Read the model definition and answer for the solid it produces. Units are mm, in the model's axes. Coordinates: 2 decimals unless noted, no trailing zeros. Order: outer loops, then holes, each group sorted by start corner. A loop starts at its lowest first (then second) coordinate and runs counter-clockwise, first axis right, second up. Notation, with made-up numbers: M -25,35 L 7,35 A31 cw 7,74 Z; hole C -28,57 d7. An arc over 180 degrees is marked long. Put each result on its own line as item: value.
from build123d import *

# Parameters (mm, degrees)
F0_R     = 17.5
F1_DEPTH = 11
F2_R     = 7.5
F3_DEPTH = 11.001
F4_R     = 0.5
F5_R     = 0.5


with BuildPart() as f1:
    # F0 (on Top) → F1 (new body)
    with BuildSketch(Plane.XY):
        Circle(F0_R)
    extrude(amount=F1_DEPTH)

    # F2 (on face) → F3 (cut, through all)
    with BuildSketch(Plane.XY.offset(11)):
        Circle(F2_R)
    extrude(amount=-F3_DEPTH, mode=Mode.SUBTRACT)

    # F4
    f4_edges = [f1.edges().sort_by_distance(p)[0] for p in [
        (-17.5, 0, 11),
        (-17.5, 0, 0),
    ]]
    fillet(f4_edges, radius=F4_R)

    # F5
    f5_edges = [f1.edges().sort_by_distance(p)[0] for p in [
        (-7.5, 0, 11),
        (-7.5, 0, 0),
    ]]
    fillet(f5_edges, radius=F5_R)


solid = f1.part
Q1. Find section A-A on x = 0. Write down the section's boundary in (y, z).
Answers below:
outline: M -17.5,0.5 A0.5 ccw -17,0 L -8,0 A0.5 ccw -7.5,0.5 L -7.5,10.5 A0.5 ccw -8,11 L -17,11 A0.5 ccw -17.5,10.5 Z; M 7.5,0.5 A0.5 ccw 8,0 L 17,0 A0.5 ccw 17.5,0.5 L 17.5,10.5 A0.5 ccw 17,11 L 8,11 A0.5 ccw 7.5,10.5 Z
Q2. Find section C-C on z = 1.75. Write down the section's boundary in (x, y).
Answers below:
outline: C 0,0 d35; hole C 0,0 d15
Q3. Consider line 1 along Y through (x, z) = (0, 3.5); line 2 along X through (y, z) = (6, 6.75); line 3 along X through (y, z) = (0.5, 1). Determine where each line is inside the solid, lowest interval first.
Answers below:
line 1: y = -17.5 to -7.5, 7.5 to 17.5
line 2: x = -16.44 to -4.5, 4.5 to 16.44
line 3: x = -17.49 to -7.48, 7.48 to 17.49
Q4. For a pull along X with two mould halves and no side action, classify faces 1 (the face through (-13.887, -10.648, 5.43)), 2 (the face through (7.3, 4, 0)), 3 (the face through (-7.493, 0.33, 5.57)) as +X half, -X half, draft (parallel to the pull), parting line (faces both ways), or undercut.
Answers below:
face 1: parting line
face 2: draft
face 3: undercut
Q5. Given pin 1 (5 mm diameter, centred on y = 4, z = 7, fed in from -X); pin 2 (10 mm diameter, centred on x = -1, y = 9.5, fed in from -Z); pin 3 (1 mm diameter, centred on x = 6, z = 4, fed in from -Y); pin 4 (1 mm diameter, centred on y = 8, z = 6, fed in from +X), each flat-ended and moving along its own axis, determine where each tip first touches the part or whether it passes through.
Answers below:
pin 1: stops at x = -17.44
pin 2: stops at z = 0
pin 3: stops at y = -16.61
pin 4: stops at x = 15.81
